Geometry: final body of the model. Coordinates: model frame, mm. Round coordinates to 2 decimals unless told otherwise and drop trailing zeros. Write each loop counter-clockwise with the first axis right and the second up, starting at its lowest first coordinate (ties: lowest second). Pieces come first, ordered by that corner, then holes. Notation, with made-up numbers: (38.5, -29.5) - (56.5, -29.5) arc R36 cw to (56.5, 6.5) - close; hole circle Ø3 at (-27, 35.5). An arc over 180 degrees is marked (long way). Write each question's results on one line, items separated by ' | '.
Autodesk Inventor part; units mm, degrees
ref_plane "YZ Plane" through (0, 0, 0) normal (1, 0, 0) x (0, 1, 0)
ref_plane "XZ Plane" through (0, 0, 0) normal (0, 1, 0) x (-1, 0, 0)
ref_plane "XY Plane" through (0, 0, 0) normal (0, 0, 1) x (1, 0, 0)
sketch "Sketch1" plane through (0, 0, 0) normal (0, 0, 1) x (1, 0, 0)
  line L0 (-30, 10) -> (30, 10)
  line L1 (30, 10) -> (30, -10)
  line L2 (30, -10) -> (-30, -10)
  line L3 (-30, -10) -> (-30, 10)
  line L4 (-30, 10) -> (30, -10) construction
  line L5 (30, 10) -> (-30, -10) construction
  circle A0 centre (18, 0) radius 7.5
  circle A1 centre (-18, 0) radius 7.5
  line L6 (0, 10) -> (0, -10) construction
  point P0 (0, 0)
  point P1 (0, 0)
  dimension "d0" = 60
  dimension "d1" = 20
  dimension "d2" = 15
  dimension "d3" = 36
extrude "Plate1" add sketch "Sketch1" along normal blind 2
fillet "Corner Round1" radius 6 4 edges at (-30, 10, 1) (-30, -10, 1) (30, 10, 1) (30, -10, 1)
equation "\"d4\" = Thickness"
equation "\"BendRadius\" = Thickness"
equation "\"BendReliefWidth\" = Thickness"
equation "\"BendReliefDepth\" = 0.5 * Thickness"
equation "\"CornerReliefSize\" = 4 * Thickness"
equation "\"MinimumRemnant\" = 2 * Thickness"
equation "\"TransitionRadius\" = BendRadius"
equation "\"JacobiRadiusSize\" = BendRadius"
equation "\"GapSize\" = Thickness"
properties part number "motor pillar 2"
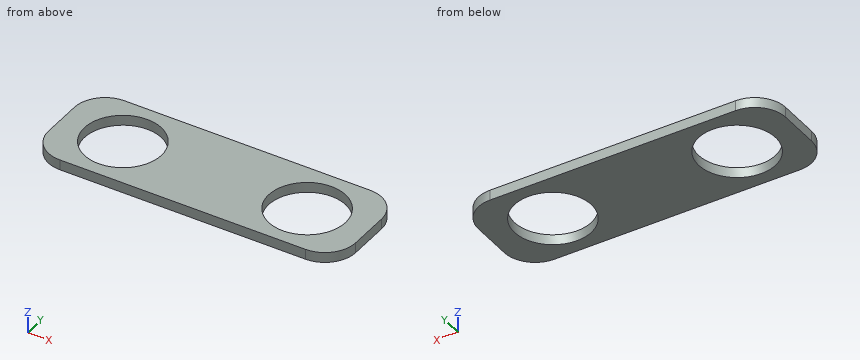
Q1. Section query C-C, the plane z = 1.7. Return loops of the section in (x, y), plus the area to 3 significant figures.
Answer block:
outline: (-30, -4) arc R6 ccw to (-24, -10) - (24, -10) arc R6 ccw to (30, -4) - (30, 4) arc R6 ccw to (24, 10) - (-24, 10) arc R6 ccw to (-30, 4) - close; hole circle Ø15 at (-18, 0); hole circle Ø15 at (18, 0) | area: 816 mm2
Q2. Section query D-D, the plane x = -17. Return loops of the section in (y, z).
Answer block:
outline: (-10, 0) - (-7.43, 0) - (-7.43, 2) - (-10, 2) - close; (7.43, 0) - (10, 0) - (10, 2) - (7.43, 2) - close
Q3. Ray query, line 1 along X through (y, z) = (2, 0.85); line 2 along X through (y, z) = (6.75, 0.8); line 3 along Y through (x, z) = (-18, 0.5). Return the intervals inside material, ascending.
Answer block:
line 1: -30 to -25.23, -10.77 to 10.77, 25.23 to 30 | line 2: -29.33 to -21.27, -14.73 to 14.73, 21.27 to 29.33 | line 3: -10 to -7.5, 7.5 to 10
Q4. Section query A-A, the plane y = 0. Return loops of the section in (x, z).
Answer block:
outline: (-30, 0) - (-25.5, 0) - (-25.5, 2) - (-30, 2) - close; (-10.5, 0) - (10.5, 0) - (10.5, 2) - (-10.5, 2) - close; (25.5, 0) - (30, 0) - (30, 2) - (25.5, 2) - close
Q5. Section query B-B, the plane x = 18. Return loops of the section in (y, z), plus the area to 3 significant figures.
Answer block:
outline: (-10, 0) - (-7.5, 0) - (-7.5, 2) - (-10, 2) - close; (7.5, 0) - (10, 0) - (10, 2) - (7.5, 2) - close | area: 10.0 mm2
